from build123d import *

# Parameters (mm, degrees)
PAD_DEPTH            = 40
PAD001_DEPTH         = 4
PAD001_DEPTH_BACK    = 3
FILLET_R             = 2
FILLET001_R          = 4
FILLET002_R          = 4
SKETCH_R             = 1.65
HOLE_DEPTH           = 32.501
SKETCH003_R          = 1.65
HOLE001_DEPTH        = 18.251
POCKET_DEPTH         = 1
POCKET_DEPTH_BACK    = 2
SKETCH005_R          = 2.8
POCKET001_DEPTH      = 1
POCKET001_DEPTH_BACK = 2
POCKET002_DEPTH      = 3


with BuildPart() as part:
    # Sketch001 → Pad (new body)
    with BuildSketch(Plane(origin=(0, 0, -5), x_dir=(1, 0, 0), z_dir=(0, 0, -1))):
        with BuildLine():
            ThreePointArc((12.5, -11.25), (18.286744, -8.983492), (22, -4))
            Line((22, -1), (22, -4))
            Line((32, -1), (22, -1))
            Line((32, -4), (32, -1))
            Line((32, -4), (25, -4))
            ThreePointArc((12.5, -14.25), (20.336868, -11.060205), (25, -4))
            Line((-12.5, -14.25), (12.5, -14.25))
            ThreePointArc((-25, -4), (-20.336868, -11.060205), (-12.5, -14.25))
            Line((-25, -4), (-25, 4))
            ThreePointArc((-23, 11.25), (-24.490833, 7.760402), (-25, 4))
            ThreePointArc((-23, 11.25), (-23.58374, 12.662164), (-24.994208, 13.249992))
            ThreePointArc((-25, 14.25), (-25.468866, 13.747264), (-24.994208, 13.249992))
            Line((-12.5, 14.25), (-25, 14.25))
            Line((12.5, 14.25), (-12.5, 14.25))
            Line((12.5, 14.25), (25, 14.25))
            ThreePointArc((24.994208, 13.249992), (25.468866, 13.747264), (25, 14.25))
            ThreePointArc((24.994208, 13.249992), (23.58374, 12.662164), (23, 11.25))
            ThreePointArc((25, 4), (24.490833, 7.760402), (23, 11.25))
            Line((32, 4), (25, 4))
            Line((32, 4), (32, 1))
            Line((32, 1), (22, 1))
            Line((22, 1), (22, 4))
            ThreePointArc((22, 4), (18.286744, 8.983492), (12.5, 11.25))
            Line((-12.5, 11.25), (12.5, 11.25))
            ThreePointArc((-12.5, 11.25), (-18.286744, 8.983492), (-22, 4))
            Line((-22, -4), (-22, 4))
            ThreePointArc((-22, -4), (-18.286744, -8.983492), (-12.5, -11.25))
            Line((-12.5, -11.25), (12.5, -11.25))
        make_face()
    extrude(amount=PAD_DEPTH)

    # Sketch002 (on Face3 of Pad) → Pad001 (join, two sides)
    with BuildSketch(Plane(origin=(0.023182, 14.25, -24), x_dir=(0, 0, 1), z_dir=(0, 1, 0))) as pad001_sk:
        with BuildLine():
            ThreePointArc((36.675, 12.664876), (38.335534, 20.835534), (30.164876, 19.175))
            ThreePointArc((27.383802, 17.3), (29.060852, 17.812531), (30.164876, 19.175))
            Line((-27.383801, 17.3), (27.383802, 17.3))
            ThreePointArc((-30.164876, 19.175), (-29.060852, 17.812531), (-27.383801, 17.3))
            ThreePointArc((-30.164876, 19.175), (-38.335534, 20.835534), (-36.675, 12.664876))
            ThreePointArc((-34.8, 9.883801), (-35.312531, 11.560852), (-36.675, 12.664876))
            Line((-34.8, -9.883801), (-34.8, 9.883801))
            ThreePointArc((-36.675, -12.664876), (-35.312531, -11.560852), (-34.8, -9.883801))
            ThreePointArc((-36.675, -12.664876), (-38.335534, -20.835534), (-30.164876, -19.175))
            ThreePointArc((-27.383801, -17.3), (-29.060852, -17.812531), (-30.164876, -19.175))
            Line((27.383801, -17.3), (-27.383801, -17.3))
            ThreePointArc((30.164876, -19.175), (29.060852, -17.812531), (27.383801, -17.3))
            ThreePointArc((30.164876, -19.175), (38.335534, -20.835534), (36.675, -12.664876))
            ThreePointArc((34.8, -9.883802), (35.312531, -11.560852), (36.675, -12.664876))
            Line((34.8, 9.883801), (34.8, -9.883802))
            ThreePointArc((36.675, 12.664876), (35.312531, 11.560852), (34.8, 9.883801))
        make_face()
    extrude(amount=PAD001_DEPTH)
    extrude(pad001_sk.sketch, amount=-PAD001_DEPTH_BACK)

    # Fillet
    fillet_edges = [part.edges().sort_by_distance(p)[0] for p in [
        (25, 4, -25),
        (25, -4, -25),
    ]]
    fillet(fillet_edges, radius=FILLET_R)

    # Fillet001
    fillet001_edges = [part.edges().sort_by_distance(p)[0] for p in [
        (32, -2.5, -45),
        (32, 2.5, -45),
        (32, 2.5, -5),
        (32, -2.5, -5),
    ]]
    fillet(fillet001_edges, radius=FILLET001_R)

    # Fillet002
    fillet002_edges = [part.edges().sort_by_distance(p)[0] for p in [
        (17.323182, 12.95802, -25),
        (-17.276818, 12.979586, -25),
    ]]
    fillet(fillet002_edges, radius=FILLET002_R)

    # Sketch (on Face29 of Pad001) → Hole (cut, through all)
    with BuildSketch(Plane(origin=(0, 18.25, -5), x_dir=(1, 0, 0), z_dir=(0, 1, 0))):
        with Locations((17.323182, -15.8)):
            Circle(SKETCH_R)
        with Locations((-17.276818, -15.8)):
            Circle(SKETCH_R)
        with Locations((17.323182, 53.8)):
            Circle(SKETCH_R)
        with Locations((-17.276818, 53.8)):
            Circle(SKETCH_R)
    extrude(amount=-HOLE_DEPTH, mode=Mode.SUBTRACT)

    # Sketch003 (on Face56 of Hole) → Hole001 (cut, through all)
    with BuildSketch(Plane(origin=(0, 4, -5), x_dir=(1, 0, 0), z_dir=(0, 1, 0))):
        with Locations((28, 30)):
            Circle(SKETCH003_R)
        with Locations((28, 10)):
            Circle(SKETCH003_R)
    extrude(amount=-HOLE001_DEPTH, mode=Mode.SUBTRACT)

    # Sketch004 (on Face25 of Hole001) → Pocket (cut, two sides)
    with BuildSketch(Plane(origin=(0, -4, -5), x_dir=(-1, 0, 0), z_dir=(0, -1, 0))) as pocket_sk:
        Polygon((-30.71066, 31.565), (-30.71066, 28.435), (-28, 26.87), (-25.28934, 28.435), (-25.28934, 31.565), (-28, 33.13), align=None)
        Polygon((-28, 13.13), (-30.71066, 11.565), (-30.71066, 8.435), (-28, 6.87), (-25.28934, 8.435), (-25.28934, 11.565), align=None)
    extrude(amount=-POCKET_DEPTH, mode=Mode.SUBTRACT)
    extrude(pocket_sk.sketch, amount=POCKET_DEPTH_BACK, mode=Mode.SUBTRACT)

    # Sketch005 (on Face66 of Pocket) → Pocket001 (cut, two sides)
    with BuildSketch(Plane(origin=(0, 4, -5), x_dir=(1, 0, 0), z_dir=(0, 1, 0))) as pocket001_sk:
        with Locations((28, 30)):
            Circle(SKETCH005_R)
        with Locations((28, 10)):
            Circle(SKETCH005_R)
    extrude(amount=-POCKET001_DEPTH, mode=Mode.SUBTRACT)
    extrude(pocket001_sk.sketch, amount=POCKET001_DEPTH_BACK, mode=Mode.SUBTRACT)

    # Sketch006 (on Face8 of Pocket001) → Pocket002 (cut)
    with BuildSketch(Plane(origin=(0, 11.25, -5), x_dir=(-1, 0, 0), z_dir=(0, -1, 0))):
        Polygon((20.406818, -15.8), (18.841818, -13.08934), (15.711818, -13.08934), (14.146818, -15.8), (15.711818, -18.51066), (18.841818, -18.51066), align=None)
        Polygon((-14.193182, -15.8), (-15.758182, -13.08934), (-18.888182, -13.08934), (-20.453182, -15.8), (-18.888182, -18.51066), (-15.758182, -18.51066), align=None)
        Polygon((20.406818, 53.8), (18.841818, 56.51066), (15.711818, 56.51066), (14.146818, 53.8), (15.711818, 51.08934), (18.841818, 51.08934), align=None)
        Polygon((-14.193182, 53.8), (-15.758182, 56.51066), (-18.888182, 56.51066), (-20.453182, 53.8), (-18.888182, 51.08934), (-15.758182, 51.08934), align=None)
    extrude(amount=-POCKET002_DEPTH, mode=Mode.SUBTRACT)


solid = part.part
Here's how the part is built. I have some questions about the finished solid (model axes, mm). A direction names the side the tool comes from. Give positions to 0.01 mm unless a question says otherwise; leave off trailing zeros. Loops run counter-clockwise (first coordinate to the right, second up) from the corner with the lowest first, then second, coordinate; pieces in that order, holes last. Notation, with made-up numbers: (37, 11.25) -> (87, 11.25) arc R21 cw to (87, 18.25) -> close; hole circle Ø1 at (29.5, 39.5). An arc over 180 degrees is marked (long way). One line per item, written item: value.
Q1. If I drill on line 1 along X through (y, z) = (1.95, -15); line 2 along Y through (x, z) = (-6.5, -30); line 3 along Z through (x, y) = (28, 3.5), over which ranges is the centre line in solid material (lowest first)?
Answers follow:
line 1: -25 to -22, 22 to 26.35, 29.65 to 32
line 2: -14.25 to -11.25, 11.25 to 18.25
line 3: -45 to -37.8, -32.2 to -17.8, -12.2 to -5
Q2. Suppose I cut it at A-A on x = -7. Please give me the cut outline in (y, z), then the cut area to 3 significant figures.
Answers follow:
outline: (-14.25, -45) -> (-11.25, -45) -> (-11.25, -5) -> (-14.25, -5) -> close; (11.25, -58.8) -> (18.25, -58.8) -> (18.25, 10.8) -> (11.25, 10.8) -> close
area: 607 mm^2
Q3. I'm going to push flat-ended pins straight in: pin 1 Ø5 at (x, z) = (28.5, -32) entering from -Y; pin 2 Ø1 at (x, y) = (-19.5, 7.5) entering from -Z; pin 3 Ø3 at (x, y) = (-15, 7.5) entering from -Z; pin 4 Ø1 at (x, z) = (-19.5, -9) entering from +Y. Where does each tip first touch, or does it pass through?
Answers follow:
pin 1: y = -4.2
pin 2: z = -45
pin 3: through
pin 4: y = 12.04
Q4. We'd pull the mould along Z, two halves only. Please class faces 5 (the face through (-18.925, 16.278, 10.727)), 6 (the face through (18.897, 16.278, 10.304)), 7 (the face through (-11.52, 14.8, 11.3)), 8 (the face through (25.316, 4.337, -25.28)): pulls with the +Z half, pulls with the -Z half, needs draft (parallel to the pull), parting line crosses it, or undercut.
Answers follow:
face 5: undercut
face 6: undercut
face 7: pulls with the +Z half
face 8: needs draft
Q5. Suppose I cut it at B-B on y = -7.5. Please give me the cut outline in (x, z), then the cut area to 3 significant figures.
Answers follow:
outline: (-24.56, -45) -> (-19.88, -45) -> (-19.88, -5) -> (-24.56, -5) -> close; (19.88, -45) -> (24.56, -45) -> (24.56, -5) -> (19.88, -5) -> close
area: 374 mm^2
Q6. Suppose I cut it at C-C on z = -15. State how many separate pieces and enclosed holes the cut face has, then the cut area to 3 significant figures.
Answers follow:
separate pieces: 3
enclosed holes: 0
area: 586 mm^2
Q7. On a 3-axis mill with a long thin cutter (end or side, diameter ignored), from which of +Z, -Z, +X, -X, +Y, -Y can I reach the whole of each face in a straight line? I mean faces 1 (the face through (28, 3, -33)), 2 (the face through (17.8, 13.4, -24.7)), 3 (the face through (25.54, -4.51, -25.28)), 4 (the face through (-19.6, 12.7, 12.2)). Say none if no direction works.
Answers follow:
face 1: +Y
face 2: +X, +Y
face 3: +Z, -Z, +X
face 4: -Y
